Verification items for the finished model (mm, model axes). A direction names the side the tool comes from. Coordinates: 2 decimals unless noted, no trailing zeros. Order: outer loops, then holes, each group sorted by start corner. A loop starts at its lowest first (then second) coordinate and runs counter-clockwise, first axis right, second up. Notation, with made-up numbers: (24.25, 83.5) -> (73.25, 83.5) arc R24 cw to (73.25, 96.5) -> close; hole circle Ø9 at (-19.5, 47.25). An arc over 180 degrees is marked (long way). Write item = value, one per line. Start each with the question number.
1. Set-up check for faces 1 (the flat face through (0, 0.2, 2)), 2 (the flat face through (0, 0, 2)): record each of +Z, -Z, +X, -X, +Y, -Y from which the full face is reachable in a straight line by a thin tool's end or side.
2. Go/stop test with flat-tipped pins: P1, Ø1, axis at x = -2, y = 2.5, coming from the +Z side; P2, Ø1, axis at x = -3, y = 8.5, coming from the -Z side; P3, Ø4, axis at x = -1, z = 7, coming from the -Y side. Record where each tip stops, or that it passes through.
3. Cross-section at C-C on z = 12.5. Record the cut outline in (x, y).
4. Thickness scan on line 1 along X through (y, z) = (12.5, 6.5); line 2 along Y through (x, z) = (3.75, 1.5); line 3 along Z through (x, y) = (3.5, 7.75). Record the ranges inside material, lowest first. Write a range as from..to.
5. Cross-section at D-D on y = 13. Record the cut outline in (x, z), plus the area to 3 significant figures.
6. Cross-section at B-B on x = 1. Record the cut outline in (y, z), plus the area to 3 significant figures.
7. Release check for a two-part mould opening along X. For faces 3 (the flat face through (0, 21, 7)), 4 (the flat face through (0, 11, 0)), 5 (the flat face through (8.1, 10, 7)), 6 (the flat face through (0, 11, 0.2)) record: +X half, -X half, draft (parallel to the pull), parting line (faces both ways), or undercut.
8. Cross-section at A-A on x = -5. Record the cut outline in (y, z).
from build123d import *

# Parameters (mm, degrees)
BOX040_W     = 12.8
BOX040_H     = 0.2
BOX040_DEPTH = 9.6
BOX041_W     = 4.2
BOX041_H     = 0.2
BOX041_DEPTH = 1.6
BOX007_W     = 15.8
BOX007_H     = 20.8
BOX007_DEPTH = 13.2
FILLET008_R  = 0.1
BOX039_W     = 16.2
BOX039_H     = 21.2
BOX039_DEPTH = 13.4
FILLET011_R  = 0.3


with BuildPart() as cube032:
    # Box040 → Box040 (new body)
    with BuildSketch(Plane(origin=(-6.4, 0, 2.2), x_dir=(1, 0, 0), z_dir=(0, 0, 1))):
        with Locations((6.4, 0.1)):
            Rectangle(BOX040_W, BOX040_H)
    extrude(amount=BOX040_DEPTH)


with BuildPart() as cube033:
    # Box041 → Box041 (new body)
    with BuildSketch(Plane(origin=(-2.1, 0, 11.8), x_dir=(1, 0, 0), z_dir=(0, 0, 1))):
        with Locations((2.1, 0.1)):
            Rectangle(BOX041_W, BOX041_H)
    extrude(amount=BOX041_DEPTH)


with BuildPart() as fusion042:
    # Box007 → Box007 (new body)
    with BuildSketch(Plane(origin=(-7.9, 0.2, 0.2), x_dir=(1, 0, 0), z_dir=(0, 0, 1))):
        with Locations((7.9, 10.4)):
            Rectangle(BOX007_W, BOX007_H)
    extrude(amount=BOX007_DEPTH)

    # Fillet008
    fillet008_edges = [fusion042.edges().sort_by_distance(p)[0] for p in [
        (-7.9, 0.2, 6.8),
        (-7.9, 21, 6.8),
        (-7.9, 10.6, 0.2),
        (7.9, 0.2, 6.8),
        (7.9, 21, 6.8),
        (7.9, 10.6, 0.2),
        (0, 0.2, 0.2),
        (0, 21, 0.2),
    ]]
    fillet(fillet008_edges, radius=FILLET008_R)

    # Fusion042: union Cube032, Cube033
    add(cube032.part)
    add(cube033.part)


with BuildPart() as shield001:
    # Box039 → Box039 (new body)
    with BuildSketch(Plane(origin=(-8.1, 0, 0), x_dir=(1, 0, 0), z_dir=(0, 0, 1))):
        with Locations((8.1, 10.6)):
            Rectangle(BOX039_W, BOX039_H)
    extrude(amount=BOX039_DEPTH)

    # Fillet011
    fillet011_edges = [shield001.edges().sort_by_distance(p)[0] for p in [
        (-8.1, 0, 6.7),
        (-8.1, 21.2, 6.7),
        (-8.1, 10.6, 0),
        (8.1, 0, 6.7),
        (8.1, 21.2, 6.7),
        (8.1, 10.6, 0),
        (0, 0, 0),
        (0, 21.2, 0),
    ]]
    fillet(fillet011_edges, radius=FILLET011_R)

    # Cut009: cut Fusion042
    add(fusion042.part, mode=Mode.SUBTRACT)


solid = shield001.part
Worked out:
q1.face_1 = +Z
q1.face_2 = +Z, -Z, +X, -X, -Y
q2.P1 = 0.2
q2.P2 = 0
q2.P3 = 21
q3.outline = (-8.1, 0.3) arc R0.3 ccw to (-7.8, 0) -> (-2.1, 0) -> (-2.1, 0.2) -> (-7.8, 0.2) arc R0.1 cw to (-7.9, 0.3) -> (-7.9, 20.9) arc R0.1 cw to (-7.8, 21) -> (7.8, 21) arc R0.1 cw to (7.9, 20.9) -> (7.9, 0.3) arc R0.1 cw to (7.8, 0.2) -> (2.1, 0.2) -> (2.1, 0) -> (7.8, 0) arc R0.3 ccw to (8.1, 0.3) -> (8.1, 20.9) arc R0.3 ccw to (7.8, 21.2) -> (-7.8, 21.2) arc R0.3 ccw to (-8.1, 20.9) -> close
q4.line_1 = -8.1..-7.9, 7.9..8.1
q4.line_2 = 0..0.2, 21..21.2
q4.line_3 = 0..0.2
q5.outline = (-8.1, 0.3) arc R0.3 ccw to (-7.8, 0) -> (7.8, 0) arc R0.3 ccw to (8.1, 0.3) -> (8.1, 13.4) -> (7.9, 13.4) -> (7.9, 0.3) arc R0.1 cw to (7.8, 0.2) -> (-7.8, 0.2) arc R0.1 cw to (-7.9, 0.3) -> (-7.9, 13.4) -> (-8.1, 13.4) -> close
q5.area = 8.49 mm²
q6.outline = (0, 0.3) arc R0.3 ccw to (0.3, 0) -> (20.9, 0) arc R0.3 ccw to (21.2, 0.3) -> (21.2, 13.4) -> (21, 13.4) -> (21, 0.3) arc R0.1 cw to (20.9, 0.2) -> (0.3, 0.2) arc R0.1 cw to (0.2, 0.3) -> (0.2, 2.2) -> (0, 2.2) -> close
q6.area = 7.25 mm²
q7.face_3 = undercut
q7.face_4 = draft
q7.face_5 = +X half
q7.face_6 = undercut
q8.outline = (0, 0.3) arc R0.3 ccw to (0.3, 0) -> (20.9, 0) arc R0.3 ccw to (21.2, 0.3) -> (21.2, 13.4) -> (21, 13.4) -> (21, 0.3) arc R0.1 cw to (20.9, 0.2) -> (0.3, 0.2) arc R0.1 cw to (0.2, 0.3) -> (0.2, 2.2) -> (0, 2.2) -> close; (0, 11.8) -> (0.2, 11.8) -> (0.2, 13.4) -> (0, 13.4) -> close
